Autodesk Inventor part; units mm, degrees
ref_plane "YZ Plane" through (0, 0, 0) normal (1, 0, 0) x (0, 1, 0)
ref_plane "XZ Plane" through (0, 0, 0) normal (0, 1, 0) x (-1, 0, 0)
ref_plane "XY Plane" through (0, 0, 0) normal (0, 0, 1) x (1, 0, 0)
sketch "Skizze1" plane through (0, 0, 0) normal (0, 1, 0) x (-1, 0, 0)
  line L0 (54.5, 0) -> (61, 0)
  line L1 (61, 0) -> (61, -32.7433)
  arc A0 (55.25, -44.0542) -> (61, -32.7433) centre (47, -32.7433) ccw
  arc A1 (55.25, -44.0542) -> (49.5, -55.3652) centre (63.5, -55.3652) ccw
  line L2 (54.5, 0) -> (54.5, -2.9933)
  line L3 (54.5, -2.9933) -> (56.5, -2.9933)
  line L4 (56.5, -2.9933) -> (56.5, -21.9933)
  line L5 (56.5, -21.9933) -> (54.5, -21.9933)
  arc A2 (6.5, -21.9933) -> (54.5, -21.9933) centre (30.5, -21.9933) ccw
  arc A3 (11.5, -55.3652) -> (5.75, -44.0542) centre (-2.5, -55.3652) ccw
  arc A4 (0, -32.7433) -> (5.75, -44.0542) centre (14, -32.7433) ccw
  line L6 (0, -32.7433) -> (0, 0)
  line L7 (0, 0) -> (6.5, 0)
  line L8 (6.5, 0) -> (6.5, -2.9933)
  line L9 (6.5, -2.9933) -> (4.5, -2.9933)
  line L10 (4.5, -2.9933) -> (4.5, -21.9933)
  line L11 (4.5, -21.9933) -> (6.5, -21.9933)
  line L12 (11.5, -55.3652) -> (11.5, -61.3652)
  line L13 (11.5, -61.3652) -> (49.5, -61.3652)
  line L14 (49.5, -61.3652) -> (49.5, -55.3652)
  line L15 (49.5, -55.3652) -> (49.5, -61.3652)
  line L16 (30.5, -51.8632) -> (30.5, -31.0026) construction
  point P0 (54.5, -1.4967)
  point P1 (6.5, -1.4967)
  point P2 (30.5, -21.9933)
  point P3 (30.5, -61.3652)
  point P4 (56.5, -12.4933)
  dimension "d2" = 2
  dimension "d3" = 19
  dimension "d4" = 14
  dimension "d5" = 14
  dimension "d6" = 38
  dimension "d10" = 19
  dimension "d12" = 2
  dimension "d13" = 24
  dimension "d14" = 24
  dimension "d18" = 4.5
  dimension "d19" = 4.5
  dimension "d20" = 24
  dimension "d54" = 19
  dimension "d55" = 6
  dimension "d56" = 14
  dimension "d57" = 14
  dimension "d58" = 42.8719
  dimension "d59" = 10.75
extrude "Extrusion1" add sketch "Skizze1" along normal blind 12
sketch "Skizze2" plane through (-11.5, 0, -61.3652) normal (0, 0, -1) x (-1, 0, 0)
  line L0 (0, 0) -> (0, 12)
  line L1 (0, 0) -> (38, 0)
  point P0 (-11.5, 0)
  point P1 (6.5, 6)
  point P2 (31.5, 6)
  point P3 (0, 6)
  point P4 (19, 0)
  dimension "d35" = 25
  dimension "d36" = 12.5
hole "Bohrung1" at (-18, 6, -61.3652) at (-43, 6, -61.3652) direction (0, 0, 1) diameter 4.134 end through all
sketch "Skizze3" plane through (0, 0, 0) normal (1, 0, 0) x (0, 0, -1)
  line L0 (0, 0) -> (0, 12)
  point P0 (12.5, 6)
  point P1 (0, 6)
  dimension "d44" = 12.5
hole "Bohrung2" at (0, 6, -12.5) direction (1, 0, 0) diameter 6 depth 4.5
sketch "Skizze4" plane through (-61, 0, -32.7433) normal (-1, 0, 0) x (0, 0, 1)
  line L0 (32.7433, 0) -> (32.7433, 12)
  point P0 (20.2433, 6)
  point P1 (32.7433, 6)
  dimension "d53" = 12.5
hole "Bohrung3" at (-61, 6, -12.5) direction (1, 0, 0) diameter 6 end through all
equation "\"d10\" = d3"
equation "\"d19\" = d18"
properties part number "102"
Read the model definition and answer for the solid it produces. Units are mm, in the model's axes. A direction names the side the tool comes from. Coordinates: 2 decimals unless noted, no trailing zeros. Loops run counter-clockwise (first coordinate to the right, second up) from the corner with the lowest first, then second, coordinate; pieces in that order, holes last. Notation, with made-up numbers: (-1.5, -16) -> (9.5, -16) arc R16 ccw to (9.5, 13) -> close; hole circle Ø7 at (-12, 17). An arc over 180 degrees is marked (long way). Answer in a Markdown table with one row per item.
Item 1: Straight lines are drawn through the part: line 1 along Y through (x, z) = (-18, -49.25); line 2 along X through (y, z) = (9, -16); line 3 along X through (y, z) = (7, -42.5). For each, find the intervals that lie inside material, in ascending order. Write a range as [from, to].
Returned:
| item | result |
|---|---|
| line 1 | y = [0, 3.93], [8.07, 12] |
| line 2 | x = [-61, -56.5], [-4.5, 0] |
| line 3 | x = [-57.04, -44.81], [-16.19, -3.96] |
Item 2: A cutting plane is placed at C-C on z = -35.5. Determine the outline of the cut face in (x, y), plus the area to 3 significant figures.
Returned:
| item | result |
|---|---|
| outline | (-60.73, 0) -> (-50.34, 0) -> (-50.34, 12) -> (-60.73, 12) -> close; (-10.66, 0) -> (-0.27, 0) -> (-0.27, 12) -> (-10.66, 12) -> close |
| area | 249 mm^2 |
Item 3: A cutting plane is placed at B-B on x = -43. Determine the outline of the cut face in (y, z).
Returned:
| item | result |
|---|---|
| outline | (0, -61.37) -> (3.93, -61.37) -> (3.93, -42.48) -> (0, -42.48) -> close; (8.07, -61.37) -> (12, -61.37) -> (12, -42.48) -> (8.07, -42.48) -> close |
Item 4: A cutting plane is placed at A-A on z = -12.5. Determine the outline of the cut face in (x, y).
Returned:
| item | result |
|---|---|
| outline | (-61, 0) -> (-56.5, 0) -> (-56.5, 3) -> (-61, 3) -> close; (-61, 9) -> (-56.5, 9) -> (-56.5, 12) -> (-61, 12) -> close; (-4.5, 0) -> (0, 0) -> (0, 3) -> (-4.5, 3) -> close; (-4.5, 9) -> (0, 9) -> (0, 12) -> (-4.5, 12) -> close |
Item 5: Each of these flat-tipped pins is pushed along its axis until it touches: P1, Ø3.5, axis at x = -43, y = 6, coming from the -Z side; P2, Ø5, axis at y = 3.5, z = -57, coming from the +X side; P3, Ø0.6, axis at x = -5.5, y = 7.5, coming from the -Z side; P4, Ø0.6, axis at x = -56, y = 3, coming from the -Z side. Where does it stop, or does it pass through?
Returned:
| item | result |
|---|---|
| P1 | passes through |
| P2 | stops at x = -11.47 |
| P3 | stops at z = -44.09 |
| P4 | stops at z = -43.71 |
Item 6: For faces 5 (the flat face through (-11.5, 6, -58)), 6 (the flat face through (0, 6, -17)), 7 (the flat face through (-54.5, 6, -1)), 8 (the flat face through (-56.5, 3, -10)), determine the directions among +Z, -Z, +X, -X, +Y, -Y from which every point of the face is accessible in a straight line to the end or side of a thin tool.
Returned:
| item | result |
|---|---|
| face 5 | -Z, +X, +Y, -Y |
| face 6 | +Z, -Z, +X, +Y, -Y |
| face 7 | +Z, +Y, -Y |
| face 8 | +Y, -Y |
Item 7: For a pull along Y with two mould halves and no side action, classify faces 1 (the flat face through (-6.5, 6, -1)), 2 (the cylindrical face through (-58.72, 3.97, -14.71)), 3 (the flat face through (-28, 0, -49)), 4 (the cylindrical face through (-2.22, 3.97, -14.71)) as released by +Y, released by -Y, zero draft, split by the parting line, or undercut.
Returned:
| item | result |
|---|---|
| face 1 | zero draft |
| face 2 | undercut |
| face 3 | released by -Y |
| face 4 | undercut |
Item 8: A cutting plane is placed at D-D on z = -50. Determine the outline of the cut face in (x, y).
Returned:
| item | result |
|---|---|
| outline | (-50.57, 0) -> (-10.43, 0) -> (-10.43, 12) -> (-50.57, 12) -> close; hole circle Ø4.13 at (-43, 6); hole circle Ø4.13 at (-18, 6) |
